The listing builds one solid part. Answer for the finished solid, in the listing's coordinates (mm). Round coordinates to 2 decimals unless told otherwise and drop trailing zeros. Loops run counter-clockwise (first coordinate to the right, second up) from the corner with the lowest first, then second, coordinate; pieces in that order, holes last. Notation, with made-up numbers: (24.25, 29) -> (56.25, 29) arc R14 ccw to (56.25, 46) -> close; hole circle Ø4 at (11, 83). An arc over 180 degrees is marked (long way). One line per question, with ' | ' between items.
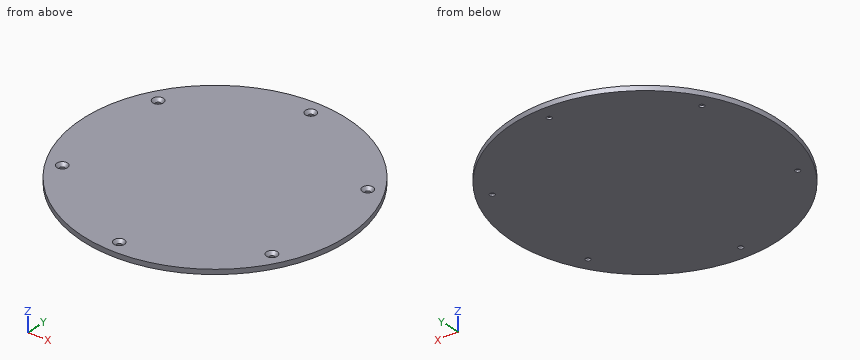
from build123d import *

# Parameters (mm, degrees)
SKETCH1_R           = 82.5
SKETCH1_R_2         = 1.5
BOSS_EXTRUDE1_DEPTH = 3
CHAMFER1_SIZE       = 1.8


with BuildPart() as part:
    # Sketch1 → Boss-Extrude1 (new body)
    with BuildSketch(Plane.XY):
        Circle(SKETCH1_R)
        with Locations((0, 74)):
            Circle(SKETCH1_R_2, mode=Mode.SUBTRACT)
        with Locations((0, -74)):
            Circle(SKETCH1_R_2, mode=Mode.SUBTRACT)
        with Locations((64.08587988, 37)):
            Circle(SKETCH1_R_2, mode=Mode.SUBTRACT)
        with Locations((64.08587988, -37)):
            Circle(SKETCH1_R_2, mode=Mode.SUBTRACT)
        with Locations((-64.08587988, -37)):
            Circle(SKETCH1_R_2, mode=Mode.SUBTRACT)
        with Locations((-64.08587988, 37)):
            Circle(SKETCH1_R_2, mode=Mode.SUBTRACT)
    extrude(amount=BOSS_EXTRUDE1_DEPTH)

    # Chamfer1
    chamfer1_edges = [part.edges().sort_by_distance(p)[0] for p in [
        (62.58587988, 37, 3),
        (62.58587988, -37, 3),
        (-65.58587988, -37, 3),
        (-65.58587988, 37, 3),
        (-1.5, 74, 3),
        (-1.5, -74, 3),
    ]]
    chamfer(chamfer1_edges, length=CHAMFER1_SIZE)


solid = part.part
Q1. A cutting plane is placed at A-A on z = 0.7. Give the vertices of the cut face in (x, y).
Numbers:
outline: circle Ø165 at (0, 0); hole circle Ø3 at (-64.09, -37); hole circle Ø3 at (-64.09, 37); hole circle Ø3 at (0, -74); hole circle Ø3 at (0, 74); hole circle Ø3 at (64.09, -37); hole circle Ø3 at (64.09, 37)
Q2. A cutting plane is placed at C-C on x = -40.5. Give the vertices of the cut face in (y, z).
Numbers:
outline: (-71.87, 0) -> (71.87, 0) -> (71.87, 3) -> (-71.87, 3) -> close
Q3. Find the intervals of material crossed by line 1 (Y direction, x = 0, z = 0.85); line 2 (X direction, y = 36.5, z = 2); line 3 (X direction, y = -38, z = 1.9), in increasing order. Write a range as from..to.
Numbers:
line 1: -82.5..-75.5, -72.5..72.5, 75.5..82.5 | line 2: -73.99..-66.33, -61.84..61.84, 66.33..73.99 | line 3: -73.23..-66.05, -62.13..62.13, 66.05..73.23
Q4. Given pin 1 Ø1 at (y, z) = (36.5, 2.5) entering from -X; pin 2 Ø5 at (x, y) = (24.5, -25.5) entering from -Z; pin 3 Ø1.8 at (x, y) = (0, -74) entering from +Z; pin 4 Ø5 at (x, y) = (-64.09, 37) entering from +Z, each flat-ended and moving along its own axis, determine where each tip first touches the part or whether it passes through.
Numbers:
pin 1: x = -74.23 | pin 2: z = 0 | pin 3: through | pin 4: z = 2.2
Q5. A cutting plane is placed at B-B on y = -31. Give the vertices of the cut face in (x, z).
Numbers:
outline: (-76.45, 0) -> (76.45, 0) -> (76.45, 3) -> (-76.45, 3) -> close
